The model under review builds one solid part; all positions refer to its coordinate system, in mm. Give positions to 0.01 mm unless a question says otherwise; leave off trailing zeros. Order: outer loops, then holes, each group sorted by start corner. A loop starts at its lowest first (then second) coordinate and runs counter-clockwise, first axis right, second up. Notation, with made-up numbers: (-25.5, 12.5) - (20.5, 12.5) arc R20 ccw to (20.5, 23.5) - close; hole circle Ø9 at (5.5, -27.5). An arc over 180 degrees is marked (long way). Write item = value, one per line. Start each with the question number.
1. We need section B-B, the plane x = 33. Give the boundary of the cut face in (y, z) (3 decimals), and give its area (3 significant figures).
2. We need section C-C, the plane y = 164.5. Give the boundary of the cut face in (x, z) (3 decimals), and give its area (3 significant figures).
3. Wall thickness on probe 1 along X at (y, z) = (103, 2.95); probe 2 along X at (y, z) = (135, 0.4); probe 3 along Y at (x, z) = (152, 0.7): over which ranges is each line inside the solid? List them lowest first.
4. We need section D-D, the plane y = 95. Give the boundary of the cut face in (x, z) (3 decimals), and give its area (3 significant figures).
5. For P1, Ø1, axis at x = 84, z = 1.5, coming from the +Y side; P2, Ø1.6, axis at y = 8, z = 2, coming from the -X side; P3, Ø1.6, axis at x = 132.5, z = 2.5, coming from the +Y side; P4, Ø10, axis at x = 151, y = 86.5, coming from the -Z side, all flat-tipped, find the tip position at first contact; note any pin that passes through.
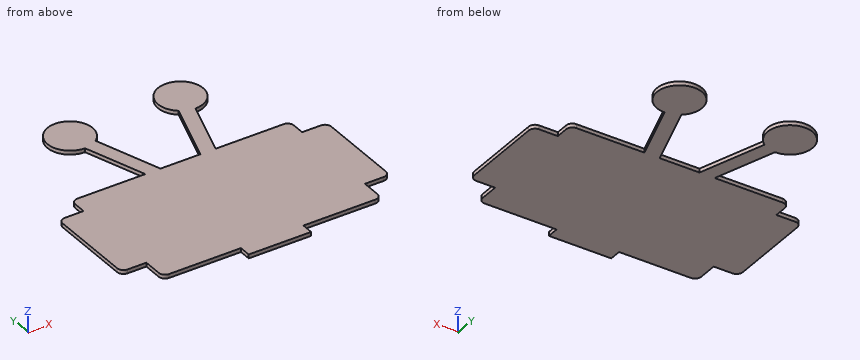
from build123d import *

# Parameters (mm, degrees)
BOSS_EXTRUDE1_DEPTH = 3.175


with BuildPart() as part:
    # Sketch1 → Boss-Extrude1 (new body)
    with BuildSketch(Plane.XY):
        with BuildLine():
            Line((0, -5.08), (58.42, -5.08))
            Line((58.42, -5.08), (58.42, -14.605))
            Line((58.42, -14.605), (109.22, -14.605))
            Line((109.22, -14.605), (109.22, -5.08))
            Line((109.22, -5.08), (167.64, -5.08))
            ThreePointArc((167.64, -5.08), (171.232102448, -3.592102448), (172.72, 0))
            Line((172.72, 0), (172.72, 15.24))
            Line((172.72, 15.24), (187.96, 15.24))
            ThreePointArc((187.96, 15.24), (191.552102448, 16.727897552), (193.04, 20.32))
            Line((193.04, 20.32), (193.04, 87.2236))
            ThreePointArc((193.04, 87.2236), (191.552102448, 90.815702448), (187.96, 92.3036))
            Line((187.96, 92.3036), (172.72, 92.3036))
            Line((172.72, 92.3036), (172.72, 102.4636))
            ThreePointArc((172.72, 102.4636), (171.232102448, 106.055702448), (167.64, 107.5436))
            Line((167.64, 107.5436), (112.428072163, 107.5436))
            Line((112.428072163, 107.5436), (128.760921922, 156.912121991))
            ThreePointArc((128.760921922, 156.912121991), (134.645312677, 192.644346081), (117.613615035, 160.685948618))
            Line((117.613615035, 160.685948618), (100.032250213, 107.5436))
            Line((100.032250213, 107.5436), (67.607749787, 107.5436))
            Line((67.607749787, 107.5436), (50.026384965, 160.685948618))
            ThreePointArc((50.026384965, 160.685948618), (32.994687323, 192.644346081), (38.879078078, 156.912121991))
            Line((38.879078078, 156.912121991), (55.211927837, 107.5436))
            Line((55.211927837, 107.5436), (0, 107.5436))
            ThreePointArc((0, 107.5436), (-3.592102448, 106.055702448), (-5.08, 102.4636))
            Line((-5.08, 102.4636), (-5.08, 92.3036))
            Line((-5.08, 92.3036), (-20.32, 92.3036))
            ThreePointArc((-20.32, 92.3036), (-23.912102448, 90.815702448), (-25.4, 87.2236))
            Line((-25.4, 87.2236), (-25.4, 20.32))
            ThreePointArc((-25.4, 20.32), (-23.912102448, 16.727897552), (-20.32, 15.24))
            Line((-20.32, 15.24), (-5.08, 15.24))
            Line((-5.08, 15.24), (-5.08, 0))
            ThreePointArc((-5.08, 0), (-3.592102448, -3.592102448), (0, -5.08))
        make_face()
    extrude(amount=BOSS_EXTRUDE1_DEPTH)


solid = part.part
Model answer:
q1.outline = (-5.08, 0) - (107.544, 0) - (107.544, 3.175) - (-5.08, 3.175) - close; (157.879, 0) - (192.646, 0) - (192.646, 3.175) - (157.879, 3.175) - close
q1.area = 468 mm2
q2.outline = (24.016, 0) - (53.742, 0) - (53.742, 3.175) - (24.016, 3.175) - close; (113.898, 0) - (143.624, 0) - (143.624, 3.175) - (113.898, 3.175) - close
q2.area = 189 mm2
q3.probe_1 = -5.05 to 172.69
q3.probe_2 = 46.13 to 58.52, 109.12 to 121.51
q3.probe_3 = -5.08 to 107.54
q4.outline = (-5.08, 0) - (172.72, 0) - (172.72, 3.175) - (-5.08, 3.175) - close
q4.area = 565 mm2
q5.P1 = 107.54
q5.P2 = -5.08
q5.P3 = 193.38
q5.P4 = 0
